```python
from build123d import *

# Parameters (mm, degrees)
F1_DEPTH = 76.2
F2_R     = 14.9020196794
F3_DEPTH = 30.48
F4_R     = 20.9265916745
F5_DEPTH = 26.162
F6_W     = 18.0814868103
F6_H     = 45.72
F6_W_2   = 10.3915287182
F6_H_2   = 19.3799102616
F7_DEPTH = 4.572
F8_R     = 7.2599789629
F9_DEPTH = 110.998


with BuildPart() as f1:
    # F0 (on Front) → F1 (new body)
    with BuildSketch(Plane.XZ):
        Polygon((9.0407434051, 27.8245471418), (-9.0407434051, 27.8245471418), (-23.6689735182, 17.1965158552), (-29.2564602261, 0), (-23.6689735182, -17.1965158552), (-9.0407434051, -27.8245471418), (9.0407434051, -27.8245471418), (23.6689735182, -17.1965158552), (29.2564602261, 0), (23.6689735182, 17.1965158552), align=None)
    extrude(amount=F1_DEPTH)

    # F2 (on face) → F3 (cut)
    with BuildSketch(Plane.XZ.offset(76.2)):
        Polygon((29.2564602261, 0), (23.6689735182, 17.1965158552), (9.0407434051, 27.8245471418), (-9.0407434051, 27.8245471418), (-23.6689735182, 17.1965158552), (-29.2564602261, 0), (-23.6689735182, -17.1965158552), (-9.0407434051, -27.8245471418), (9.0407434051, -27.8245471418), (23.6689735182, -17.1965158552), align=None)
        Circle(F2_R, mode=Mode.SUBTRACT)
    extrude(amount=-F3_DEPTH, mode=Mode.SUBTRACT)

    # F4 (on Front) → F5 (join)
    with BuildSketch(Plane.XZ):
        Circle(F4_R)
    extrude(amount=-F5_DEPTH)

    # F6 (on face) → F7 (cut)
    with BuildSketch(Plane(origin=(16.3548584617, 0, 22.5105314985), x_dir=(0.8090169944, 0, -0.5877852523), z_dir=(0.5877852523, 0, 0.8090169944))):
        with Locations((0, -22.86)):
            Rectangle(F6_W, F6_H)
        with Locations((0, -22.86)):
            Rectangle(F6_W_2, F6_H_2, mode=Mode.SUBTRACT)
    extrude(amount=-F7_DEPTH, mode=Mode.SUBTRACT)

    # F8 (on face) → F9 (cut)
    with BuildSketch(Plane(origin=(0, 26.162, 0), x_dir=(-1, 0, 0), z_dir=(0, 1, 0))):
        Circle(F8_R)
    extrude(amount=-F9_DEPTH, mode=Mode.SUBTRACT)


solid = f1.part
```
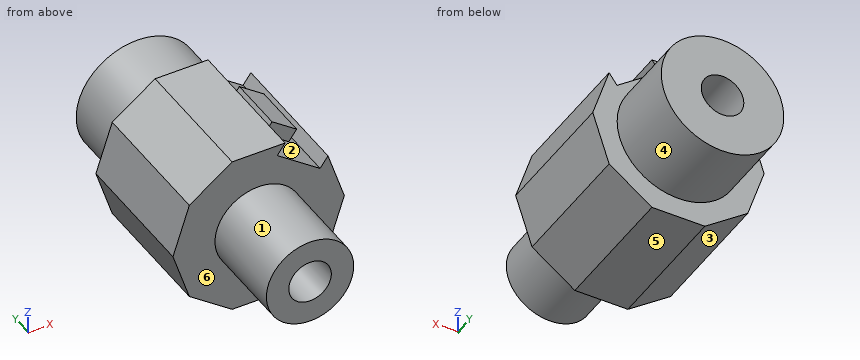
Check sheet for the modelled part. Datum: model origin and axes. Units: mm. Face numbers are marked on the shaded views. A direction names the side the tool comes from. Coordinates: 2 decimals unless noted, no trailing zeros. Write each loop counter-clockwise with the first axis right and the second up, starting at its lowest first coordinate (ties: lowest second). Pieces come first, ordered by that corner, then holes. Notation, with made-up numbers: (-31.75, 4.5) - (1.25, 4.5) arc R11 ccw to (1.25, 9.5) - close; hole circle Ø5 at (70.25, -10.75). An arc over 180 degrees is marked (long way). One line per question, with ' | ' between items.
Item 1: Thickness scan on line 1 (Z direction, x = 0, y = -50); line 2 (Z direction, x = 0, y = -17); line 3 (Y direction, x = 17, z = -21). Record the ranges inside material, lowest first. Write a range as [from, to].
Determined:
line 1: z = [-14.9, -7.26], [7.26, 14.9] | line 2: z = [-27.82, -7.26], [7.26, 27.82] | line 3: y = [-45.72, 0]
Item 2: Mould release check, pull along Z, two halves, no side actions. Record for the marked faces 1, 2 and 3: pulls with the +Z half, pulls with the -Z half, needs draft (parallel to the pull), parting line crosses it, or undercut.
Determined:
face 1: parting line crosses it | face 2: undercut | face 3: pulls with the -Z half
Item 3: Gauge pin test, flat ends, axial feed: P1, Ø1, axis at y = -64, z = 5, coming from the +X side; P2, Ø1, axis at y = 9, z = -9, coming from the -X side; P3, Ø5, axis at y = -27, z = -17, coming from the -X side; P4, Ø19, axis at x = 0, z = 0, coming from the +Y side. Record the tip position at first contact, or that the pin passes through.
Determined:
P1: stops at x = 14.21 | P2: stops at x = -19.12 | P3: stops at x = -24.55 | P4: stops at y = 26.16
Item 4: Sectioned sample at B-B on y = -39.5. Record the boundary of the cut face in (x, z), plus the area to 3 significant figures.
Determined:
outline: (-29.26, 0) - (-23.67, -17.2) - (-9.04, -27.82) - (9.04, -27.82) - (23.67, -17.2) - (29.26, 0) - (23.67, 17.2) - (20.98, 13.5) - (6.35, 24.13) - (9.04, 27.82) - (-9.04, 27.82) - (-23.67, 17.2) - close; hole circle Ø14.52 at (0, 0) | area: 2,270 mm2
Item 5: Sectioned sample at A-A on x = 0. Record the boundary of the cut face in (y, z), plus the area to 3 significant figures.
Determined:
outline: (-76.2, -14.9) - (-45.72, -14.9) - (-45.72, -27.82) - (0, -27.82) - (0, -20.93) - (26.16, -20.93) - (26.16, -7.26) - (-76.2, -7.26) - close; (-76.2, 7.26) - (26.16, 7.26) - (26.16, 20.93) - (0, 20.93) - (0, 27.82) - (-45.72, 27.82) - (-45.72, 14.9) - (-76.2, 14.9) - close | area: 3,060 mm2
Item 6: Access from +Z, -Z, +X, -X, +Y, -Y to the whole of each face (thin tool, end or side, straight path). Record for the marked faces 4, 5 and 6.
Determined:
face 4: +Y | face 5: -Z, +X, -X, +Y, -Y | face 6: -Y
Item 7: Sectioned sample at D-D on x = -16. Record the boundary of the cut face in (y, z).
Determined:
outline: (-45.72, -22.77) - (0, -22.77) - (0, -13.49) - (26.16, -13.49) - (26.16, 13.49) - (0, 13.49) - (0, 22.77) - (-45.72, 22.77) - close
Item 8: Sectioned sample at C-C on z = 3.5. Record the boundary of the cut face in (x, y), plus the area to 3 significant figures.
Determined:
outline: (-28.12, -45.72) - (-14.49, -45.72) - (-14.49, -76.2) - (-6.36, -76.2) - (-6.36, 26.16) - (-20.63, 26.16) - (-20.63, 0) - (-28.12, 0) - close; (6.36, -76.2) - (14.49, -76.2) - (14.49, -45.72) - (28.12, -45.72) - (28.12, 0) - (20.63, 0) - (20.63, 26.16) - (6.36, 26.16) - close | area: 3,230 mm2
